The listing builds one solid part. Answer for the finished solid, in the listing's coordinates (mm). A direction names the side the tool comes from. Round coordinates to 2 decimals unless told otherwise and drop trailing zeros. Write each loop counter-clockwise with the first axis right and the second up, starting at its lowest first coordinate (ties: lowest second). Pieces come first, ordered by that corner, then holes. Notation, with made-up numbers: M 69.5,85 L 114.5,85 A31 ccw 114.5,109 Z; hole C -4.5,82.5 d1. An arc over 180 degrees is marked long. One line per item, written item: value. Start each with the question number.
(1) For a pull along X with two mould halves and no side action, classify faces 1 (the cylindrical face through (-7.836, 7.79, 7.888)), 2 (the cylindrical face through (-2.75, -12.4, 7.89)), 3 (the flat face through (3, 6, 16)) as released by +X, released by -X, zero draft, split by the parting line, or undercut.
(2) Section C-C (z = 10.25) is taken. Determine the outline of the cut face in (x, y).
(3) Given P1, Ø3, axis at x = 5, z = 3, coming from the +Y side; P2, Ø8, axis at x = -7.5, z = 12, coming from the -Y side; P3, Ø2, axis at x = -3, z = 11, coming from the +Y side, each flat-ended and moving along its own axis, determine where each tip first touches the part or whether it passes through.
(4) Section A-A (x = 0) is taken. Determine the outline of the cut face in (y, z), plus the area to 3 significant figures.
(5) Consider probe 1 along X at (y, z) = (6.75, 12.25); probe 2 along Y at (x, z) = (0, 16.5); probe 3 along Z at (x, y) = (9.5, -3.5). Determine where each line is inside the solid, lowest interval first.
(6) For faces 4 (the cylindrical face through (-1.38, -6.2, 16.79)), 5 (the cylindrical face through (6.73, 7.79, 7.89)), determine the directions among +Z, -Z, +X, -X, +Y, -Y from which every point of the face is accessible in a straight line to the end or side of a thin tool.
(7) Section D-D (x = 10.25) is taken. Determine the outline of the cut face in (y, z), plus the area to 3 significant figures.
```python
from build123d import *

# Parameters (mm, degrees)
SKETCH_1_R               = 12.7
EXTRUDE_1_DEPTH          = 16
SKETCH_2_R               = 6.35
EXTRUDE_2_DEPTH          = 1.6
SKETCH_3_R               = 6.35
EXTRUDE_3_DEPTH          = 1.6
EXTRUDE_3_TAPER          = 75.857
CUT_EXTRUDE_1_DEPTH      = 25.053689946
CUT_EXTRUDE_1_DEPTH_BACK = 25.053689946
SKETCH_4_R               = 0.75
SKETCH_5_R               = 0.75
CUT_EXTRUDE_5_DEPTH      = 27.153424276


with BuildPart() as part:
    # Эскиз1 → Бобышка-Вытянуть1 (new body)
    with BuildSketch(Plane.XY):
        Circle(SKETCH_1_R)
    extrude(amount=EXTRUDE_1_DEPTH)

    # Эскиз2 → Бобышка-Вытянуть2 (add)
    with BuildSketch(Plane.XY.offset(16)):
        Circle(SKETCH_2_R)
    extrude(amount=EXTRUDE_2_DEPTH)

    # Эскиз3 → Бобышка-Вытянуть3 (add)
    with BuildSketch(Plane.XY.offset(17.6)):
        Circle(SKETCH_3_R)
    extrude(amount=EXTRUDE_3_DEPTH, taper=EXTRUDE_3_TAPER)

    # Эскиз4 → Вырез-Вытянуть1 (cut, two sides: drawn at the far end of the back side and taken through both)
    with BuildSketch(Plane.XY.offset(16).offset(-CUT_EXTRUDE_1_DEPTH_BACK)):
        Circle(SKETCH_4_R)
    extrude(amount=CUT_EXTRUDE_1_DEPTH + CUT_EXTRUDE_1_DEPTH_BACK, mode=Mode.SUBTRACT)

    # Эскиз5 → Вырез-Вытянуть5 (cut, through all)
    with BuildSketch(Plane.XY):
        with Locations((-7.283199846, 7.283199846)):
            Circle(SKETCH_5_R)
        with Locations((7.283199846, 7.283199846)):
            Circle(SKETCH_5_R)
    extrude(amount=CUT_EXTRUDE_5_DEPTH, mode=Mode.SUBTRACT)


solid = part.part
```
Recorded:
1. face 1: undercut
1. face 2: split by the parting line
1. face 3: zero draft
2. outline: C 0,0 d25.4; hole C -7.28,7.28 d1.5; hole C 0,0 d1.5; hole C 7.28,7.28 d1.5
3. P1: stops at y = 12.21
3. P2: stops at y = -12.21
3. P3: stops at y = 12.54
4. outline: M -12.7,0 L -0.75,0 L -0.75,19.01 L -6.35,17.6 L -6.35,16 L -12.7,16 Z; M 0.75,0 L 12.7,0 L 12.7,16 L 6.35,16 L 6.35,17.6 L 0.75,19.01 Z
4. area: 408 mm2
5. probe 1: x = -10.76 to -7.81, -6.76 to 6.76, 7.81 to 10.76
5. probe 2: y = -6.35 to -0.75, 0.75 to 6.35
5. probe 3: z = 0 to 16
6. face 4: +Z
6. face 5: +Z, -Z
7. outline: M -7.5,0 L 7.5,0 L 7.5,16 L -7.5,16 Z
7. area: 240 mm2
